Read the model definition and answer for the solid it produces. Units are mm, in the model's axes. Face numbers are marked on the shaded views. A direction names the side the tool comes from. Give positions to 0.01 mm unless a question says otherwise; leave off trailing zeros. Order: outer loops, then holes, each group sorted by start corner. A loop starts at its lowest first (then second) coordinate and runs counter-clockwise, first axis right, second up. Notation, with made-up numbers: M -1,28.5 L 58,28.5 A30 cw 58,58.5 Z; hole C -4,-23.75 d8. An arc over 180 degrees is marked long. One line per item, written item: value.
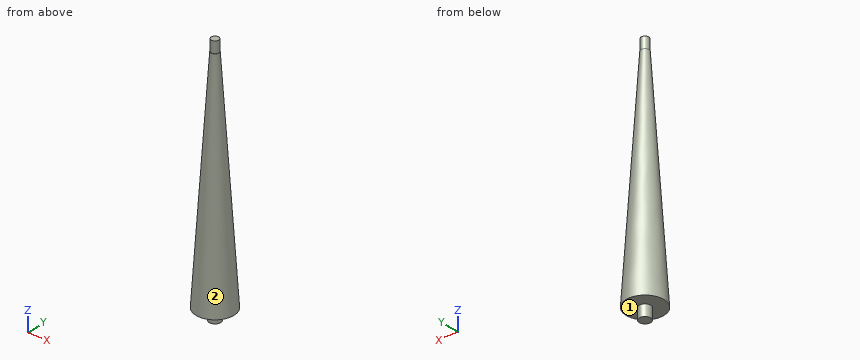
from build123d import *

# Parameters (mm, degrees)
SKETCH1_R           = 25
BOSS_EXTRUDE1_DEPTH = 300
BOSS_EXTRUDE1_TAPER = 3.75
SHELL1_T            = 5
SKETCH2_R           = 7.5
BOSS_EXTRUDE2_DEPTH = 15
SKETCH3_R           = 5
BOSS_EXTRUDE3_DEPTH = 15


with BuildPart() as part:
    # Sketch1 → Boss-Extrude1 (new body)
    with BuildSketch(Plane.XY):
        Circle(SKETCH1_R)
    extrude(amount=BOSS_EXTRUDE1_DEPTH, taper=BOSS_EXTRUDE1_TAPER)

    # Shell1 (no face opened: a closed hollow body)
    add(offset(amount=-SHELL1_T, mode=Mode.PRIVATE), mode=Mode.SUBTRACT)

    # Sketch2 → Boss-Extrude2 (add)
    with BuildSketch(Plane(origin=(0, 0, 0), x_dir=(-1, 0, 0), z_dir=(0, 0, -1))):
        Circle(SKETCH2_R)
    extrude(amount=BOSS_EXTRUDE2_DEPTH)

    # Sketch3 → Boss-Extrude3 (add)
    with BuildSketch(Plane.XY.offset(300)):
        Circle(SKETCH3_R)
    extrude(amount=BOSS_EXTRUDE3_DEPTH)


solid = part.part
1) Each of these flat-tipped pins is pushed along its axis until it touches: pin 1 Ø10 at (x, y) = (-19, 1) entering from -Z; pin 2 Ø4 at (x, z) = (7.5, 83) entering from +Y; pin 3 Ø2 at (y, z) = (8, 99.5) entering from +X. Where does it stop, or does it pass through?
Reported:
pin 1: stops at z = 0
pin 2: stops at y = 18.79
pin 3: stops at x = 17.11
2) Find section B-B, the plane z = 14. Write down the section's boundary in (x, y), plus the area to 3 significant figures.
Reported:
outline: C 0,0 d48.16; hole C 0,0 d38.14
area: 679 mm^2
3) Consider probe 1 along X at (y, z) = (15.5, 118.5); probe 2 along X at (y, z) = (-3, 159); probe 3 along Y at (x, z) = (15.5, 36.5). Determine where each line is inside the solid, lowest interval first.
Reported:
probe 1: x = -7.53 to 7.53
probe 2: x = -14.27 to -9.09, 9.09 to 14.27
probe 3: y = -16.46 to -8.33, 8.33 to 16.46
4) Which of the six approach directions +Z, -Z, +X, -X, +Y, -Y give full straight-line access (tool end or side, diameter ignored) to the marked faces 1 and 2?
Reported:
face 1: -Z
face 2: +Z
5) Find section A-A, the plane z = 250. Write down the section's boundary in (x, y).
Reported:
outline: C 0,0 d17.23; hole C 0,0 d7.21
